Design review of the part shown in the three views and the two pictorial views. Dimensions are in mm from the part's minimum x, y and z. A direction names the side the tool comes from. Give positions to 0.01 mm unless a question says otherwise; leave off trailing zeros. Loops run counter-clockwise (first coordinate to the right, second up) from the corner with the lowest first, then second, coordinate; pieces in that order, holes last.
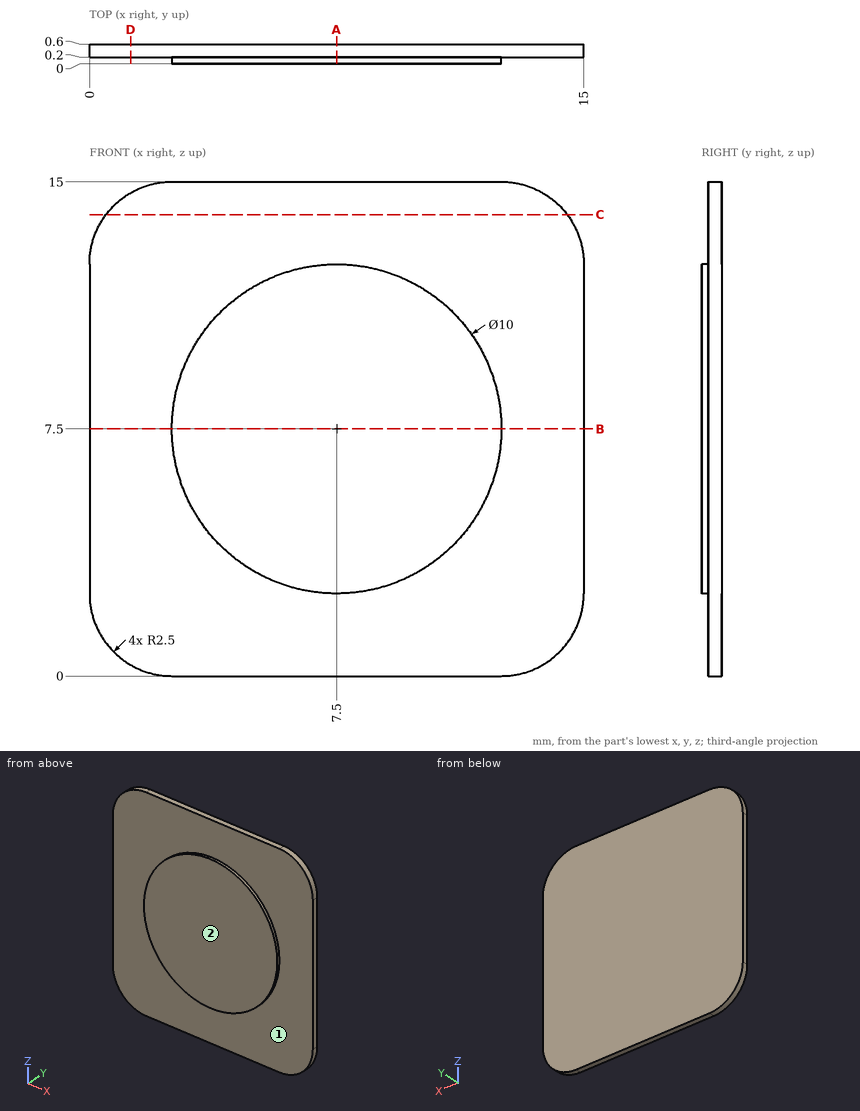
Q1. Consider section C-C on z = 14. Give the boundary of the cut face in (x, y), plus the area to 3 significant figures.
Answers:
outline: (0.5, 0.2) - (14.5, 0.2) - (14.5, 0.6) - (0.5, 0.6) - close
area: 5.60 mm2
Q2. Consider section A-A on x = 7.5. Give the boundary of the cut face in (y, z), plus the area to 3 significant figures.
Answers:
outline: (0, 2.5) - (0.2, 2.5) - (0.2, 0) - (0.6, 0) - (0.6, 15) - (0.2, 15) - (0.2, 12.5) - (0, 12.5) - close
area: 8.00 mm2
Q3. Machinability: for the marked faces 1 and 2, which of the approach directions +Z, -Z, +X, -X, +Y, -Y give a long, thin tool a straight path to every point of the face, cutting with its end or side? Answer none if there is none.
Answers:
face 1: -Y
face 2: +Z, -Z, +X, -X, -Y
Q4. Consider section D-D on x = 1.25. Give the boundary of the cut face in (y, z), plus the area to 3 significant figures.
Answers:
outline: (0.2, 0.33) - (0.6, 0.33) - (0.6, 14.67) - (0.2, 14.67) - close
area: 5.73 mm2
Q5. For probe 1 along Y at (x, z) = (0.5, 7.25); probe 2 along X at (y, z) = (0.4, 13); probe 3 along X at (y, z) = (0.05, 11.25), list the stretches that pass through material, from the lowest coordinate up.
Answers:
probe 1: y = 0.2 to 0.6
probe 2: x = 0.05 to 14.95
probe 3: x = 4.19 to 10.81
Q6. Consider section B-B on z = 7.5. Give the boundary of the cut face in (x, y).
Answers:
outline: (0, 0.2) - (2.5, 0.2) - (2.5, 0) - (12.5, 0) - (12.5, 0.2) - (15, 0.2) - (15, 0.6) - (0, 0.6) - close
